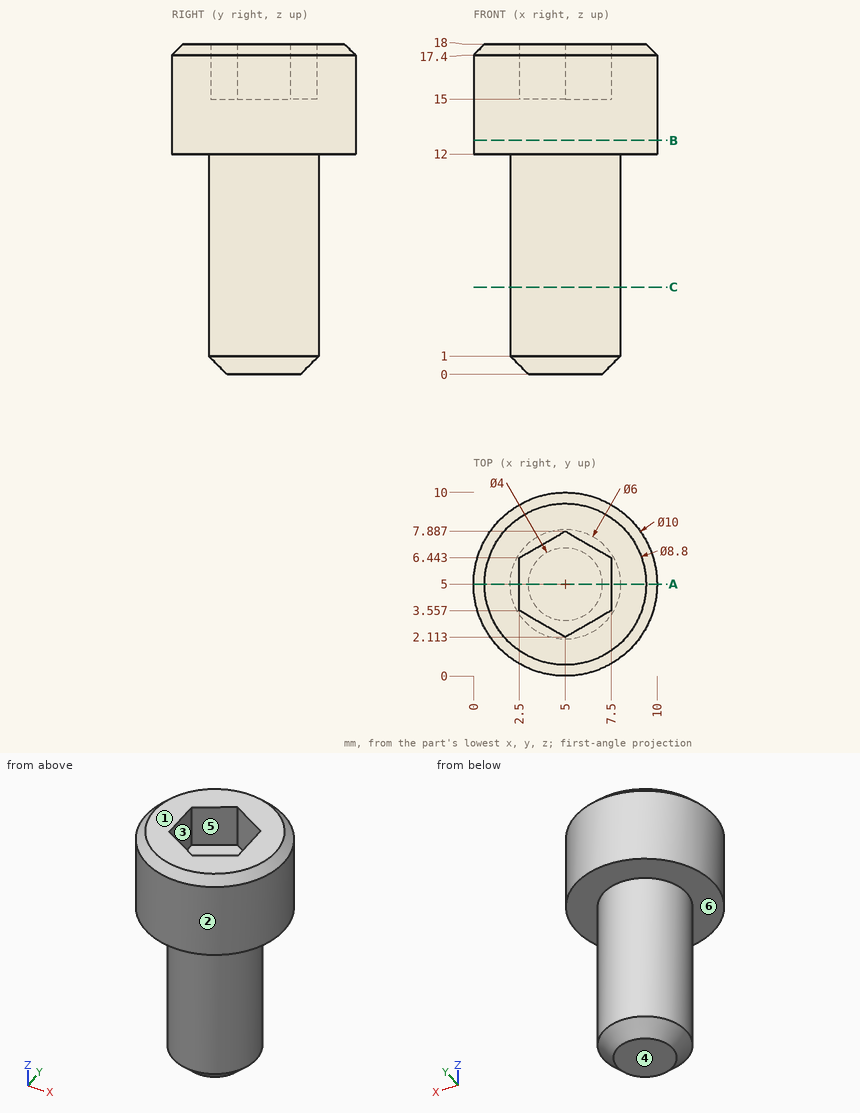
Can you work these out from the drawing? Everything is in mm from the part's minimum corner. A direction names the side the tool comes from. Give positions to 0.01 mm unless a question says otherwise; leave off trailing zeros. Write each loop counter-clockwise with the first axis right and the second up, starting at its lowest first coordinate (ties: lowest second). Pieces come first, ordered by that corner, then holes. Notation, with made-up numbers: M 63,-25 L 90,-25 A23 cw 90,-5 Z; hole C 48.25,82 d4. An arc over 180 degrees is marked long. Answer in a Markdown table with one row per item. Add a question column.
Item 1: For pin 1 Ø2 at (y, z) = (8, 14.5) entering from +X; pin 2 Ø4 at (x, y) = (5, 5.5) entering from +Z; pin 3 Ø5 at (y, z) = (1, 4) entering from +X, each with a flat end and sliding along its axis, tell me the tip position at first contact or that it passes through.
Item 2: Imagine slicing it at B-B, the plane z = 12.75. Write out the boundary of the cut face in (x, y).
Item 3: Please list where these lines run through material, in increasing order: L1, parallel to Y at x = 9, z = 12.25; L2, parallel to Z at x = 2.25, y = 8.
Item 4: We'd pull the mould along Y, two halves only. Please class the marked faces 1, 2 and 3: released by +Y, released by -Y, zero draft, split by the parting line, or undercut.
Item 5: On a 3-axis mill with a long thin cutter (end or side, diameter ignored), from which of +Z, -Z, +X, -X, +Y, -Y can I reach the whole of each face in a straight line? I mean the marked faces 4, 5 and 6. Say none if no direction works.
Item 6: Imagine slicing it at A-A, the plane y = 5. Write out the boundary of the cut face in (x, z), plus the area to 3 significant figures.
Item 7: Imagine slicing it at C-C, the plane z = 4.75. Write out the boundary of the cut face in (x, y).
Evaluation:
| question | item | result |
|---|---|---|
| 1 | pin 1 | stops at x = 9.58 |
| 1 | pin 2 | stops at z = 15 |
| 1 | pin 3 | stops at x = 7.6 |
| 2 | outline | C 5,5 d10 |
| 3 | L1 | y = 2 to 8 |
| 3 | L2 | z = 12 to 18 |
| 4 | face 1 | zero draft |
| 4 | face 2 | split by the parting line |
| 4 | face 3 | undercut |
| 5 | face 4 | -Z, +X, -X, +Y, -Y |
| 5 | face 5 | +Z |
| 5 | face 6 | -Z |
| 6 | outline | M 0,12 L 2,12 L 2,1 L 3,0 L 7,0 L 8,1 L 8,12 L 10,12 L 10,17.4 L 9.4,18 L 7.5,18 L 7.5,15 L 2.5,15 L 2.5,18 L 0.6,18 L 0,17.4 Z |
| 6 | area | 116 mm² |
| 7 | outline | C 5,5 d6 |
